Work out the finished part from the listing and answer in its coordinate system (mm). Face numbers are marked on the shaded views. A direction names the side the tool comes from. Coordinates: 2 decimals unless noted, no trailing zeros. Write each loop counter-clockwise with the first axis right and the second up, starting at its lowest first coordinate (ties: lowest second). Pieces come first, ordered by that corner, then holes. Notation, with made-up numbers: M -5.75,0 L 16.25,0 A6 ccw 16.25,5 Z; hole C 81,9 d3. An arc over 180 degrees is marked long. Use CSV: the item, a comma, the result in double quotes.
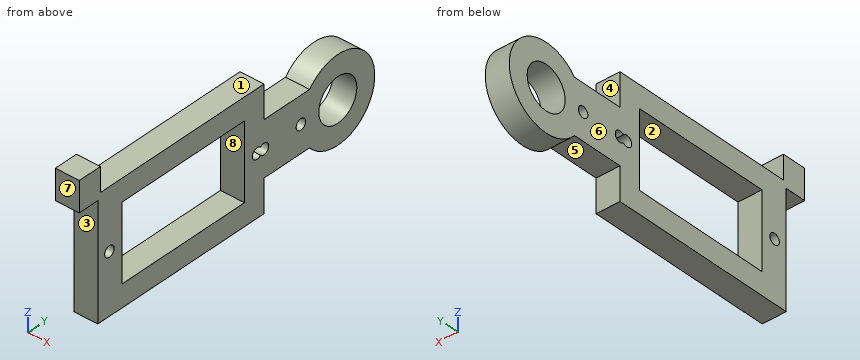
from build123d import *

# Parameters (mm, degrees)
SKETCH1_R            = 7
BOSS_EXTRUDE1_DEPTH  = 4
BOSS_EXTRUDE2_START  = -4.5
SKETCH2_W            = 4
SKETCH2_H            = 34
BOSS_EXTRUDE2_DEPTH  = 9
BOSS_EXTRUDE3_START  = -10
SKETCH3_W            = 4
SKETCH3_H            = 31.5
BOSS_EXTRUDE3_DEPTH  = 20
BOSS_EXTRUDE4_START  = 9
SKETCH4_W            = 4
SKETCH4_H            = 4
BOSS_EXTRUDE4_DEPTH  = 5
BOSS_EXTRUDE5_START  = -1
SKETCH5_R            = 3.6
BOSS_EXTRUDE5_DEPTH  = 6
BOSS_EXTRUDE6_START  = -1
SKETCH6_R            = 0.9
BOSS_EXTRUDE6_DEPTH  = 6
BOSS_EXTRUDE7_START  = -1
SKETCH7_R            = 0.9
BOSS_EXTRUDE7_DEPTH  = 6
BOSS_EXTRUDE8_START  = -6.3
SKETCH8_W            = 6
SKETCH8_H            = 23.2
BOSS_EXTRUDE8_DEPTH  = 12.6
BOSS_EXTRUDE9_START  = -1
SKETCH9_R            = 0.9
BOSS_EXTRUDE9_DEPTH  = 6
BOSS_EXTRUDE10_START = -1
SKETCH10_R           = 0.9
BOSS_EXTRUDE10_DEPTH = 6


with BuildPart() as part:
    # Sketch1 → Boss-Extrude1 (new body)
    with BuildSketch(Plane(origin=(0, 0, 0), x_dir=(0, 0, -1), z_dir=(1, 0, 0))):
        Circle(SKETCH1_R)
    extrude(amount=BOSS_EXTRUDE1_DEPTH)

    # Sketch2 → Boss-Extrude2 (add)
    with BuildSketch(Plane.XY.offset(BOSS_EXTRUDE2_START)):
        with Locations((2, -17)):
            Rectangle(SKETCH2_W, SKETCH2_H)
    extrude(amount=BOSS_EXTRUDE2_DEPTH)

    # Sketch3 → Boss-Extrude3 (add)
    with BuildSketch(Plane.XY.offset(BOSS_EXTRUDE3_START)):
        with Locations((2, -29.75)):
            Rectangle(SKETCH3_W, SKETCH3_H)
    extrude(amount=BOSS_EXTRUDE3_DEPTH)

    # Sketch4 → Boss-Extrude4 (add)
    with BuildSketch(Plane.XY.offset(BOSS_EXTRUDE4_START)):
        with Locations((2, -47)):
            Rectangle(SKETCH4_W, SKETCH4_H)
    extrude(amount=BOSS_EXTRUDE4_DEPTH)


with BuildPart() as body_2:
    # Sketch5 → Boss-Extrude5 (new body)
    with BuildSketch(Plane(origin=(0, 0, 0), x_dir=(0, 0, -1), z_dir=(1, 0, 0)).offset(BOSS_EXTRUDE5_START)):
        Circle(SKETCH5_R)
    extrude(amount=BOSS_EXTRUDE5_DEPTH)


with BuildPart() as part_1:
    add(part.part)

    # Combine1: cut body 2
    add(body_2.part, mode=Mode.SUBTRACT)


with BuildPart() as body_2_2:
    # Sketch6 → Boss-Extrude6 (new body)
    with BuildSketch(Plane(origin=(0, 0, 0), x_dir=(0, 0, -1), z_dir=(1, 0, 0)).offset(BOSS_EXTRUDE6_START)):
        with Locations((0, -7)):
            Circle(SKETCH6_R)
    extrude(amount=BOSS_EXTRUDE6_DEPTH)


with BuildPart() as part_2:
    add(part_1.part)

    # Combine2: cut body 2 2
    add(body_2_2.part, mode=Mode.SUBTRACT)


with BuildPart() as body_2_3:
    # Sketch7 → Boss-Extrude7 (new body)
    with BuildSketch(Plane(origin=(0, 0, 0), x_dir=(0, 0, -1), z_dir=(1, 0, 0)).offset(BOSS_EXTRUDE7_START)):
        with Locations((0, -14)):
            Circle(SKETCH7_R)
    extrude(amount=BOSS_EXTRUDE7_DEPTH)


with BuildPart() as part_3:
    add(part_2.part)

    # Combine3: cut body 2 3
    add(body_2_3.part, mode=Mode.SUBTRACT)


with BuildPart() as body_2_4:
    # Sketch8 → Boss-Extrude8 (new body)
    with BuildSketch(Plane.XY.offset(BOSS_EXTRUDE8_START)):
        with Locations((2, -29.3)):
            Rectangle(SKETCH8_W, SKETCH8_H)
    extrude(amount=BOSS_EXTRUDE8_DEPTH)


with BuildPart() as part_4:
    add(part_3.part)

    # Combine4: cut body 2 4
    add(body_2_4.part, mode=Mode.SUBTRACT)


with BuildPart() as body_2_5:
    # Sketch9 → Boss-Extrude9 (new body)
    with BuildSketch(Plane(origin=(0, 0, 0), x_dir=(0, 0, -1), z_dir=(1, 0, 0)).offset(BOSS_EXTRUDE9_START)):
        with Locations((0, -43.3)):
            Circle(SKETCH9_R)
    extrude(amount=BOSS_EXTRUDE9_DEPTH)


with BuildPart() as part_5:
    add(part_4.part)

    # Combine5: cut body 2 5
    add(body_2_5.part, mode=Mode.SUBTRACT)


with BuildPart() as body_2_6:
    # Sketch10 → Boss-Extrude10 (new body)
    with BuildSketch(Plane(origin=(0, 0, 0), x_dir=(0, 0, -1), z_dir=(1, 0, 0)).offset(BOSS_EXTRUDE10_START)):
        with Locations((0, -15.3)):
            Circle(SKETCH10_R)
    extrude(amount=BOSS_EXTRUDE10_DEPTH)


with BuildPart() as part_6:
    add(part_5.part)

    # Combine6: cut body 2 6
    add(body_2_6.part, mode=Mode.SUBTRACT)


solid = part_6.part
Item 1: The part is cut by section C-C (y = -15.3). Write down the section's boundary in (x, z).
Answer:
outline,"M 0,-10 L 4,-10 L 4,-0.9 L 0,-0.9 Z; M 0,0.9 L 4,0.9 L 4,10 L 0,10 Z"
Item 2: The part is cut by section D-D (x = 1.8). Write down the section's boundary in (y, z), then the cut area to 3 significant figures.
Answer:
outline,"M -49,9 L -45.5,9 L -45.5,-10 L -14,-10 L -14,-4.5 L -5.36,-4.5 A7 ccw long -5.36,4.5 L -14,4.5 L -14,10 L -45,10 L -45,14 L -49,14 Z; hole C -43.3,0 d1.8; hole M -40.9,-6.3 L -17.7,-6.3 L -17.7,6.3 L -40.9,6.3 Z; hole M -14.65,-0.62 A0.9 ccw long -14.65,0.62 A0.9 ccw long Z; hole C -7,0 d1.8; hole C 0,0 d7.2"
area,"528 mm2"
Item 3: The part is cut by section B-B (z = 0). Write down the section's boundary in (x, y), then the cut area to 3 significant figures.
Answer:
outline,"M 0,-45.5 L 4,-45.5 L 4,-44.2 L 0,-44.2 Z; M 0,-42.4 L 4,-42.4 L 4,-40.9 L 0,-40.9 Z; M 0,-17.7 L 4,-17.7 L 4,-16.2 L 0,-16.2 Z; M 0,-13.1 L 4,-13.1 L 4,-7.9 L 0,-7.9 Z; M 0,-6.1 L 4,-6.1 L 4,-3.6 L 0,-3.6 Z; M 0,3.6 L 4,3.6 L 4,7 L 0,7 Z"
area,"61.6 mm2"
Item 4: Consider probe 1 along Y at (x, z) = (1.6, 0); probe 2 along Z at (x, y) = (2.55, 0); probe 3 along Z at (x, y) = (2.8, -43.3). Determine where each line is inside the solid, lowest interval first.
Answer:
probe 1,"y = -45.5 to -44.2, -42.4 to -40.9, -17.7 to -16.2, -13.1 to -7.9, -6.1 to -3.6, 3.6 to 7"
probe 2,"z = -7 to -3.6, 3.6 to 7"
probe 3,"z = -10 to -0.9, 0.9 to 10"
Item 5: Given pin 1 (1.5 mm diameter, centred on x = 0.5, y = -30, fed in from +Z); pin 2 (1.5 mm diameter, centred on x = 3.5, z = 5.5, fed in from -Y); pin 3 (1 mm diameter, centred on x = 1, y = -47.5, fed in from -Z), each flat-ended and moving along its own axis, determine where each tip first touches the part or whether it passes through.
Answer:
pin 1,"stops at z = 10"
pin 2,"stops at y = -45.5"
pin 3,"stops at z = 9"
Item 6: For a pull along Y with two mould halves and no side action, classify the marked faces 6, 7 and 8 as released by +Y, released by -Y, zero draft, split by the parting line, or undercut.
Answer:
face 6,"zero draft"
face 7,"released by -Y"
face 8,"undercut"
Item 7: The part is cut by section A-A (y = -7). Write down the section's boundary in (x, z), then the cut area to 3 significant figures.
Answer:
outline,"M 0,-4.5 L 4,-4.5 L 4,-0.9 L 0,-0.9 Z; M 0,0.9 L 4,0.9 L 4,4.5 L 0,4.5 Z"
area,"28.8 mm2"
Item 8: A tool of negligible diameter and unlimited length cuts with its end or side. For the marked faces 1, 2, 3, 4 and 5, from which of +Z, -Z, +X, -X, +Y, -Y can it reach the whole face along a straight path? Write none if from no direction.
Answer:
face 1,"+Z, +X, -X, +Y"
face 2,"+X, -X"
face 3,"-Z, +X, -X, -Y"
face 4,"+Z, +X, -X"
face 5,"-Z, +X, -X"
